```python
from build123d import *

# Parameters (mm, degrees)
F0_W = 5
F0_H = 20
F4_D = 6


with BuildPart() as f2:
    # F2: sweep along a path in F1
    with BuildLine(Plane.XZ) as f2_path:
        Line((0, 0), (0, -55))
        ThreePointArc((0, -55), (1.4644660941, -58.5355339059), (5, -60))
        Line((5, -60), (80, -60))
    # F0 (on Top) → F2 (sweep)
    with BuildSketch(Plane.XY):
        with Locations((2.5, -10)):
            Rectangle(F0_W, F0_H)
    sweep(path=f2_path.line)

    # F4 (through all)
    with Locations(Plane.YZ.offset(5)):
        with Locations((-10, -27.5)):
            Hole(F4_D / 2)


solid = f2.part
```
Read the model definition and answer for the solid it produces. Units are mm, in the model's axes. A direction names the side the tool comes from. Coordinates: 2 decimals unless noted, no trailing zeros. Loops run counter-clockwise (first coordinate to the right, second up) from the corner with the lowest first, then second, coordinate; pieces in that order, holes last. Notation, with made-up numbers: (-38, 18.25) - (11, 18.25) arc R27 cw to (11, 46.25) - close; hole circle Ø6 at (12.5, 46.5). An arc over 180 degrees is marked (long way). Answer in a Markdown table with one row per item.
1. Determine the mould class of faces 3 (the face through (22, 0, -57)), 4 (the face through (43, -10, -60)), 5 (the face through (22, -20, -57)), 6 (the face through (2.47, -12.77, -28.65)) for opening direction Y: +Y half, -Y half, draft (parallel to the pull), parting line (faces both ways), or undercut.
Conclusion:
| item | result |
|---|---|
| face 3 | +Y half |
| face 4 | draft |
| face 5 | -Y half |
| face 6 | undercut |
2. Find section C-C, the plane y = -18.5. Write down the section's boundary in (x, z), then the cut area to 3 significant figures.
Conclusion:
| item | result |
|---|---|
| outline | (0, -55) arc R5 ccw to (5, -60) - (80, -60) - (80, -55) - (5, -55) - (5, 0) - (0, 0) - close |
| area | 670 mm² |
3. Find section B-B, the plane z = -27.5. Write down the section's boundary in (x, y), then the cut area to 3 significant figures.
Conclusion:
| item | result |
|---|---|
| outline | (0, -20) - (5, -20) - (5, -13) - (0, -13) - close; (0, -7) - (5, -7) - (5, 0) - (0, 0) - close |
| area | 70.0 mm² |
4. Find section A-A, the plane y = -10. Write down the section's boundary in (x, z).
Conclusion:
| item | result |
|---|---|
| outline | (0, -55) arc R5 ccw to (5, -60) - (80, -60) - (80, -55) - (5, -55) - (5, -30.5) - (0, -30.5) - close; (0, -24.5) - (5, -24.5) - (5, 0) - (0, 0) - close |
5. Which of the six approach directions +Z, -Z, +X, -X, +Y, -Y give full straight-line access (tool end or side, diameter ignored) to faces 1 (the face through (0, -14, -28)), 2 (the face through (5, -6, -28))?
Conclusion:
| item | result |
|---|---|
| face 1 | +Z, -Z, -X, +Y, -Y |
| face 2 | +Z, +X, +Y, -Y |
6. Find section D-D, the plane x = 15.5. Write down the section's boundary in (y, z), then the cut area to 3 significant figures.
Conclusion:
| item | result |
|---|---|
| outline | (-20, -60) - (0, -60) - (0, -55) - (-20, -55) - close |
| area | 100 mm² |
7. Given pin 1 (12 mm diameter, centred on y = -12.5, z = -44.5, fed in from +X); pin 2 (8 mm diameter, centred on x = 41, y = -14.5, fed in from +Z), each flat-ended and moving along its own axis, determine where each tip first touches the part or whether it passes through.
Conclusion:
| item | result |
|---|---|
| pin 1 | stops at x = 5 |
| pin 2 | stops at z = -55 |
8. Straight lines are drawn through the part: line 1 (X direction, y = -7.5, z = -24); line 2 (Z direction, x = 40.5, y = -11.25); line 3 (Z direction, x = 2.9, y = -10). For each, find the intervals that lie inside material, in ascending order.
Conclusion:
| item | result |
|---|---|
| line 1 | x = 0 to 5 |
| line 2 | z = -60 to -55 |
| line 3 | z = -59.54 to -30.5, -24.5 to 0 |
